For this review, use the dimensioned drawing (mm, ordinates from the lowest corner) and the shaded views. Round coordinates to 2 decimals unless told otherwise and drop trailing zeros. Loops run counter-clockwise (first coordinate to the right, second up) from the corner with the lowest first, then second, coordinate; pieces in that order, holes last. Notation, with made-up numbers: (-13.75, -11.75) - (-0.75, -11.75) arc R20 ccw to (-0.75, -4.75) - close; hole circle Ø7 at (44.5, -14.5). An arc over 180 degrees is marked (long way). Use one line per item in the form item = value. Start each with the question number.
(1) We need section B-B, the plane y = 36. Write out the cut boundary in (x, z) (3 decimals), then the cut area to 3 significant figures.
(2) We need section A-A, the plane z = 4.5. Write out the cut boundary in (x, y) (3 decimals).
(3) We need section C-C, the plane x = 5.5. Write out the cut boundary in (y, z) (3 decimals).
(4) Wall thickness on probe 1 along Y at (x, z) = (36.5, 3.75) (3 decimals); probe 2 along X at (y, z) = (37.5, 3.5) (3 decimals): over which ranges is each line inside the solid? List them lowest first. Write a range as [from, to].
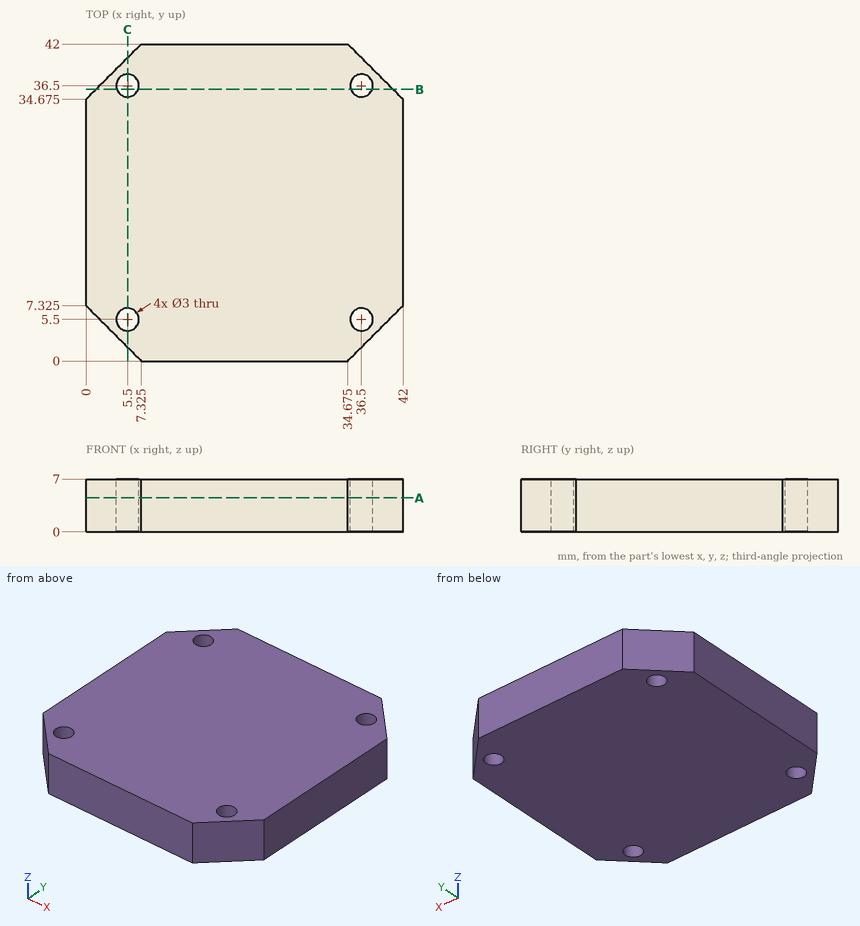
Data:
q1.outline = (1.325, 0) - (4.086, 0) - (4.086, 7) - (1.325, 7) - close; (6.914, 0) - (35.086, 0) - (35.086, 7) - (6.914, 7) - close; (37.914, 0) - (40.675, 0) - (40.675, 7) - (37.914, 7) - close
q1.area = 236 mm^2
q2.outline = (0, 7.325) - (7.325, 0) - (34.675, 0) - (42, 7.325) - (42, 34.675) - (34.675, 42) - (7.325, 42) - (0, 34.675) - close; hole circle Ø3 at (5.5, 5.5); hole circle Ø3 at (5.5, 36.5); hole circle Ø3 at (36.5, 5.5); hole circle Ø3 at (36.5, 36.5)
q3.outline = (1.825, 0) - (4, 0) - (4, 7) - (1.825, 7) - close; (7, 0) - (35, 0) - (35, 7) - (7, 7) - close; (38, 0) - (40.175, 0) - (40.175, 7) - (38, 7) - close
q4.probe_1 = [1.825, 4], [7, 35], [38, 40.175]
q4.probe_2 = [2.825, 4.382], [6.618, 35.382], [37.618, 39.175]
